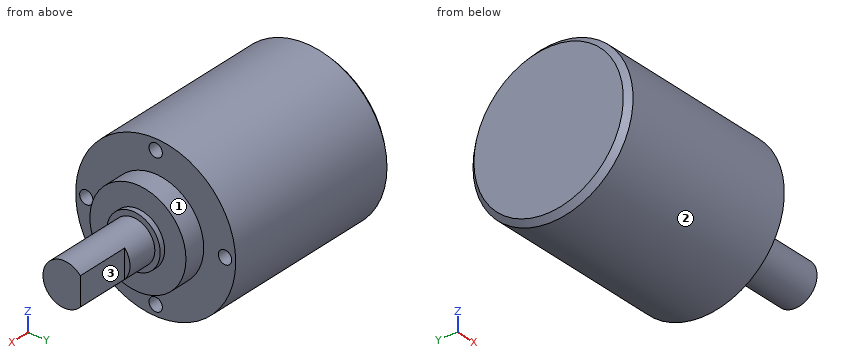
```python
from build123d import *

# Parameters (mm, degrees)
EXTRUSION1_DEPTH             = 10
R_P_TITION_CIRCULAIRE1_COUNT = 4
CHANFREIN1_SIZE              = 1


with BuildPart() as part:
    # Esquisse1 → Révolution1 (revolve)
    with BuildSketch(Plane.XY):
        Polygon((27.85, 0), (27.85, 4), (12.25, 4), (12.25, 5), (11.25, 5), (11.25, 9), (7.25, 9), (7.25, 15), (-27.85, 15), (-27.85, 0), align=None)
    revolve(axis=Axis((-27.85, 0, 0), (1, 0, 0)))

    # Esquisse2 → Extrusion1 (cut)
    with BuildSketch(Plane(origin=(27.85, 0, 0), x_dir=(0, 0, -1), z_dir=(1, 0, 0))):
        with BuildLine():
            Line((2.645751311, 3), (-2.645751311, 3))
            ThreePointArc((-2.645751311, 3), (0, 4), (2.645751311, 3))
        make_face()
    extrude(amount=-EXTRUSION1_DEPTH, mode=Mode.SUBTRACT)

    # Esquisse3 → Trou taraudé M31 (revolve, cut)
    with BuildSketch(Plane(origin=(7.25, 13, 0), x_dir=(0, 0, -1), z_dir=(0, 1, 0))):
        Polygon((0, 0), (0, 6.251075774), (1.25, 5.5), (1.25, 0), align=None)
    trou_taraud_m31 = revolve(axis=Axis((13.6, 13, 0), (-1, 0, 0)), mode=Mode.SUBTRACT)

    # Répétition circulaire1: Trou taraudé M31 ×4 about axis
    r_p_tition_circulaire1_axis = Axis((0, 0, 0), (1, 0, 0))
    for i in range(1, R_P_TITION_CIRCULAIRE1_COUNT):
        add(trou_taraud_m31.rotate(r_p_tition_circulaire1_axis, i * 360 / R_P_TITION_CIRCULAIRE1_COUNT), mode=Mode.SUBTRACT)

    # Chanfrein1
    chanfrein1_edges = [part.edges().sort_by_distance(p)[0] for p in [
        (-27.85, -15, 0),
    ]]
    chamfer(chanfrein1_edges, length=CHANFREIN1_SIZE)


solid = part.part
```
Input: part model. Units: mm. Frame: model coordinates. Face numbers are marked on the shaded views. A direction names the side the tool comes from. Round coordinates to 2 decimals unless told otherwise and drop trailing zeros. Loops run counter-clockwise (first coordinate to the right, second up) from the corner with the lowest first, then second, coordinate; pieces in that order, holes last. Notation, with made-up numbers: (61.25, 66.25) -> (106.25, 66.25) arc R24 ccw to (106.25, 87.25) -> close; hole circle Ø11 at (53.25, 46.5). An arc over 180 degrees is marked (long way). Use one line per item in the form item = value. Start each with the question number.
Item 1: Contact query for flat-ended pins moving along their axis: pin 1 Ø2.5 at (x, z) = (23, 0.5) entering from +Y; pin 2 Ø6 at (x, z) = (-21.5, -4) entering from +Y; pin 3 Ø1 at (y, z) = (8.5, -3.5) entering from +X. Output: stop coordinate, or through.
Item 2: Section query C-C on x = 21.5. Return the cut outline in (y, z).
Item 3: Section query B-B on x = -21. Return the cut outline in (y, z).
Item 4: Material intervals for L1, parallel to Z at x = 3.15, y = 0; L2, parallel to X at y = -6, z = -10.75; L3, parallel to Z at x = 3.95, y = 13, sorted ascending. Write a range as from..to.
Item 5: Set-up query: the marked faces 1, 2 and 3. Return all of +Z, -Z, +X, -X, +Y, -Y with unobstructed straight access to the full face (end or side cutting, diameter ignored); none if empty.
Item 6: Section query A-A on x = 5.5. Return the cut outline in (y, z), then the cut area to 3 significant figures.
Ans:
q1.pin_1 = 3
q1.pin_2 = 14.97
q1.pin_3 = 11.25
q2.outline = (3, -2.65) -> (3, 2.65) arc R4 ccw (long way) to start
q3.outline = circle Ø30 at (0, 0)
q4.L1 = -15..-14.25, -11.75..11.75, 14.25..15
q4.L2 = -27.85..7.25
q4.L3 = -7.48..-1.25, 1.25..7.48
q5.face_1 = +X
q5.face_2 = +X, -X
q5.face_3 = +Z, -Z, +X, +Y
q6.outline = circle Ø30 at (0, 0); hole circle Ø2.5 at (-13, 0); hole circle Ø2.5 at (0, -13); hole circle Ø2.5 at (0, 13); hole circle Ø2.5 at (13, 0)
q6.area = 687 mm^2
